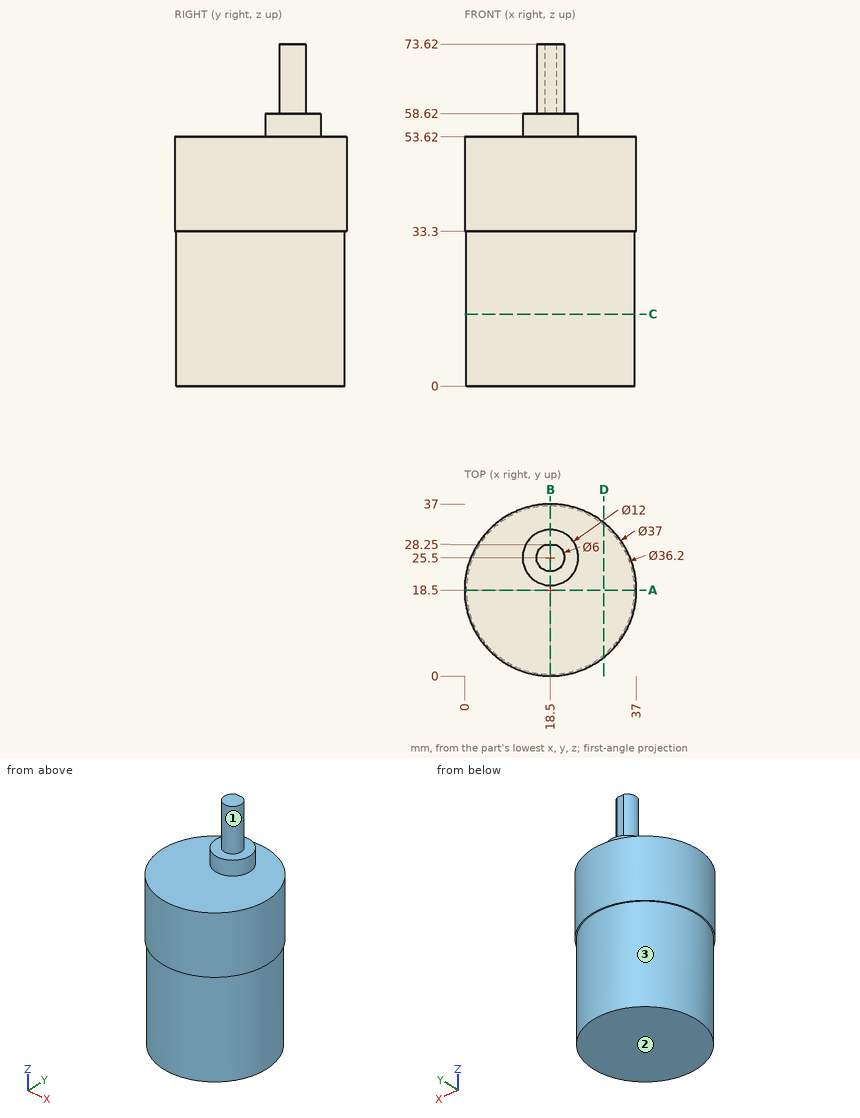
Source: three-view drawing plus pictorial views. Frame: mm from the lowest corner of the part. A direction names the side the tool comes from. Round coordinates to 2 decimals unless told otherwise and drop trailing zeros. Loops run counter-clockwise (first coordinate to the right, second up) from the corner with the lowest first, then second, coordinate; pieces in that order, holes last.
1. Section query A-A on y = 18.5. Output: boundary loops of the cut face in (x, z).
2. Section query B-B on x = 18.5. Output: boundary loops of the cut face in (y, z), and give its area (3 significant figures).
3. Section query D-D on x = 30. Output: boundary loops of the cut face in (y, z).
4. Access query for the marked faces 1, 2 and 3. Directions: +Z, -Z, +X, -X, +Y, -Y. A direction counts if a zero-diameter tool reaches every point of the face in a straight line with its end or side. Return the directions, or none.
5. Ray query, L1, parallel to Z at x = 25.5, y = 7.5; L2, parallel to X at y = 18, z = 47; L3, parallel to X at y = 2, z = 41. Return the intervals inside material, ascending.
6. Section query C-C on z = 15.5. Output: boundary loops of the cut face in (x, y), and give its area (3 significant figures).
7. Contact query for flat-ended pins moving along their axis: pin 1 (1.9 mm diameter, centred on x = 18, z = 69, fed in from +Y); pin 2 (4 mm diameter, centred on x = 17, z = 13, fed in from +Y); pin 3 (12 mm diameter, centred on x = 6, z = 47.5, fed in from +Y); pin 4 (2 mm diameter, centred on x = 8.5, y = 12, fed in from -Z). Output: stop coordinate, or through.
Answers below:
1. outline: (0, 33.3) - (0.4, 33.3) - (0.4, 0) - (36.6, 0) - (36.6, 33.3) - (37, 33.3) - (37, 53.62) - (0, 53.62) - close
2. outline: (0, 33.3) - (0.4, 33.3) - (0.4, 0) - (36.6, 0) - (36.6, 33.3) - (37, 33.3) - (37, 53.62) - (31.5, 53.62) - (31.5, 58.62) - (28.25, 58.62) - (28.25, 73.62) - (22.5, 73.62) - (22.5, 58.62) - (19.5, 58.62) - (19.5, 53.62) - (0, 53.62) - close
2. area: 2,100 mm2
3. outline: (4.01, 33.3) - (4.52, 33.3) - (4.52, 0) - (32.48, 0) - (32.48, 33.3) - (32.99, 33.3) - (32.99, 53.62) - (4.01, 53.62) - close
4. face 1: +Z
4. face 2: -Z, +X, -X, +Y, -Y
4. face 3: -Z
5. L1: z = 0 to 53.62
5. L2: x = 0.01 to 36.99
5. L3: x = 10.13 to 26.87
6. outline: circle Ø36.2 at (18.5, 18.5)
6. area: 1,030 mm2
7. pin 1: stops at y = 28.25
7. pin 2: stops at y = 36.6
7. pin 3: stops at y = 35.82
7. pin 4: stops at z = 0
